Autodesk Fusion 360 part; units mm, degrees
sketch "Sketch1" plane through (0, 0, 0) normal (0, 0, 1) x (1, 0, 0)
  circle A0 centre (0, 0) radius 48
  line L0 (9, -34) -> (-9, -34)
  line L1 (-9, -34) -> (-9, -28)
  line L2 (-9, -28) -> (9, -28)
  line L3 (9, -28) -> (9, -34)
  line L4 (9, -34) -> (-9, -28) construction
  line L5 (-9, -34) -> (9, -28) construction
  line L6 (3, -10) -> (-3, -10)
  line L7 (-3, -10) -> (-3, 0)
  line L8 (-3, 0) -> (3, 0)
  line L9 (3, 0) -> (3, -10)
  line L10 (3, -10) -> (-3, 0) construction
  line L11 (-3, -10) -> (3, 0) construction
  line L12 (-17, 6) -> (-23, 6)
  line L13 (-23, 6) -> (-23, 24)
  line L14 (-23, 24) -> (-17, 24)
  line L15 (-17, 24) -> (-17, 6)
  line L16 (-17, 6) -> (-23, 24) construction
  line L17 (-23, 6) -> (-17, 24) construction
  line L18 (23, 6) -> (17, 6)
  line L19 (17, 6) -> (17, 24)
  line L20 (17, 24) -> (23, 24)
  line L21 (23, 24) -> (23, 6)
  line L22 (23, 6) -> (17, 24) construction
  line L23 (17, 6) -> (23, 24) construction
  line L24 (0, -48) -> (0, 48) construction
  line L25 (-20, 15) -> (20, 15) construction
  point P0 (0, -31)
  point P1 (-20, 15)
  point P2 (0, -5)
  point P3 (20, 15)
  point P4 (0, -31)
  point P5 (0, -5)
  point P6 (-20, 15)
  point P7 (20, 15)
  point P8 (0, 15)
  dimension "d1" = 96
  dimension "d2" = 18
  dimension "d3" = 6
  dimension "d4" = 10
  dimension "d5" = 6
  dimension "d6" = 18
  dimension "d7" = 6
  dimension "d8" = 18
  dimension "d9" = 6
  dimension "d12" = 31
  dimension "d13" = 40
  dimension "d14" = 15
extrude "Extrude3" add sketch "Sketch1" along normal blind 3
Model file for the job. Use its own axes, mm. A direction names the side the tool comes from. Coordinates: 2 decimals unless noted, no trailing zeros. Loops run counter-clockwise (first coordinate to the right, second up) from the corner with the lowest first, then second, coordinate; pieces in that order, holes last. Notation, with made-up numbers: M -32,30.5 L -10,30.5 A24 ccw -10,43.5 Z; hole C -32,68.5 d5. An arc over 180 degrees is marked long. Use CSV: the item, a comma, the result in double quotes. Start each with the question number.
1. Tool access for faces 1 (the flat face through (-1, 1, 3)), 2 (the flat face through (20, 24, 1)): list every direction of +Z, -Z, +X, -X, +Y, -Y with a clear straight run to the whole face (end or side of a thin tool).
2. Probe probe 1 along Y at (x, z) = (1, 1.9); probe 2 along X at (y, z) = (20.5, 2.1); probe 3 along X at (y, z) = (15, 2.6). List the from-to ranges inside material, lowest first. Write a range as [from, to].
3. Flat gauge pins, fed straight in: pin 1 (0.9 mm diameter, centred on x = -0.5, z = 2, fed in from -Y); pin 2 (1 mm diameter, centred on y = -24, z = 2, fed in from -X); pin 3 (1.5 mm diameter, centred on x = 1, z = 2, fed in from +Y). Where does each tip first touch, or does it go through?
4. Band-saw the part on C-C, the plane y = 8. List the corners of the cut face in (x, z), then the cut area to 3 significant figures.
5. Band-saw the part on D-D, the plane x = 12.5. List the corners of the cut face in (y, z), then the cut area to 3 significant figures.
6. Band-saw the part on A-A, the plane x = 0. List the corners of the cut face in (y, z).
7. Band-saw the part on B-B, the plane z = 2.05. List the corners of the cut face in (x, y), then the cut area to 3 significant figures.
8. Two-plate mould, pull along Y, no slides. Class faces 3 (the flat face through (-1, 1, 0)), 4 (the cylindrical face through (-47.954, -2.11, 1.479)), 5 (the flat face through (-20, 24, 1)): pulls with the +Y half, pulls with the -Y half, needs draft (parallel to the pull), parting line crosses it, or undercut.
Entries:
1,face 1,"+Z, +X, -X, +Y, -Y"
1,face 2,"+Z, -Z"
2,probe 1,"y = [-47.99, -34], [-28, -10], [0, 47.99]"
2,probe 2,"x = [-43.4, -23], [-17, 17], [23, 43.4]"
2,probe 3,"x = [-45.6, -23], [-17, 17], [23, 45.6]"
3,pin 1,"stops at y = -48"
3,pin 2,"stops at x = -41.85"
3,pin 3,"stops at y = 48"
4,outline,"M -47.33,0 L -23,0 L -23,3 L -47.33,3 Z; M -17,0 L 17,0 L 17,3 L -17,3 Z; M 23,0 L 47.33,0 L 47.33,3 L 23,3 Z"
4,area,"248 mm2"
5,outline,"M -46.34,0 L 46.34,0 L 46.34,3 L -46.34,3 Z"
5,area,"278 mm2"
6,outline,"M -48,0 L -34,0 L -34,3 L -48,3 Z; M -28,0 L -10,0 L -10,3 L -28,3 Z; M 0,0 L 48,0 L 48,3 L 0,3 Z"
7,outline,"C 0,0 d96; hole M -23,6 L -17,6 L -17,24 L -23,24 Z; hole M -9,-34 L 9,-34 L 9,-28 L -9,-28 Z; hole M -3,-10 L 3,-10 L 3,0 L -3,0 Z; hole M 17,6 L 23,6 L 23,24 L 17,24 Z"
7,area,"6,850 mm2"
8,face 3,"needs draft"
8,face 4,"parting line crosses it"
8,face 5,"undercut"
